Job drawing, mm, ordinate dimensions from the low corner. One solid piece. Give positions to 0.01 mm unless a question says otherwise; leave off trailing zeros. Write each loop counter-clockwise with the first axis right and the second up, starting at its lowest first coordinate (ties: lowest second). Pieces come first, ordered by that corner, then holes. Notation, with made-up numbers: (1, 81.5) - (51, 81.5) arc R26 cw to (51, 110.5) - close; hole circle Ø3 at (55.25, 32). An arc over 180 degrees is marked (long way). Answer as a JSON object with one key per item and string values.
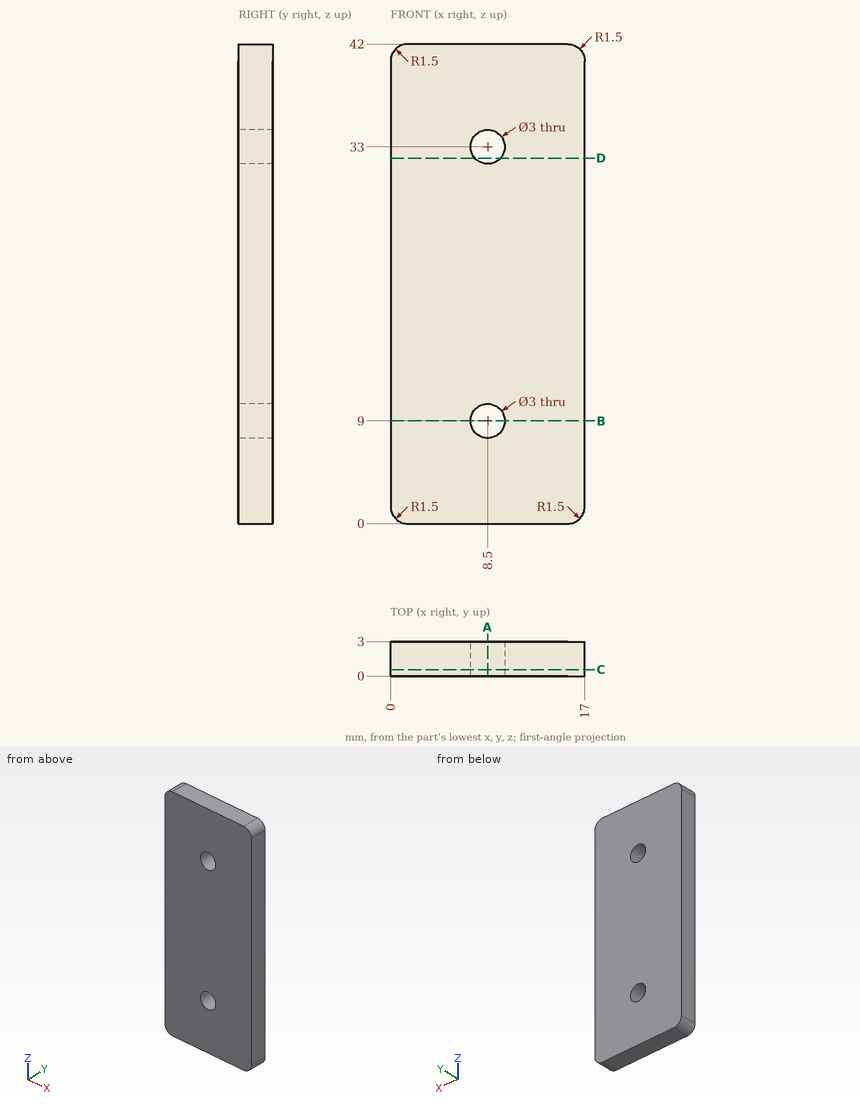
Item 1: Cut at A-A (x = 8.5). Give the cut face in (y, z), and give its area (3 significant figures).
Entries:
{"outline": "(0, 0) - (3, 0) - (3, 7.5) - (0, 7.5) - close; (0, 10.5) - (3, 10.5) - (3, 31.5) - (0, 31.5) - close; (0, 34.5) - (3, 34.5) - (3, 42) - (0, 42) - close", "area": "108 mm2"}
Item 2: Flat gauge pins, fed straight in: P1, Ø5, axis at x = 8.5, z = 9, coming from the +Y side; P2, Ø2.5, axis at x = 8.5, z = 33, coming from the -Y side. Where does each tip first touch, or does it go through?
Entries:
{"P1": "y = 3", "P2": "through"}
Item 3: Cut at D-D (z = 32). Give the cut face in (x, y), and give its area (3 significant figures).
Entries:
{"outline": "(0, 0) - (7.38, 0) - (7.38, 3) - (0, 3) - close; (9.62, 0) - (17, 0) - (17, 3) - (9.62, 3) - close", "area": "44.3 mm2"}
Item 4: Probe line 1 (Z direction, x = 8.5, y = 2); line 2 (Z direction, x = 9, y = 1.7); line 3 (X direction, y = 2.85, z = 8.5). List the from-to ranges inside material, lowest first. Write a range as from..to.
Entries:
{"line 1": "0..7.5, 10.5..31.5, 34.5..42", "line 2": "0..7.59, 10.41..31.59, 34.41..42", "line 3": "0..7.09, 9.91..17"}
Item 5: Cut at C-C (y = 0.55). Give the cut face in (x, z), and give its area (3 significant figures).
Entries:
{"outline": "(0, 1.5) arc R1.5 ccw to (1.5, 0) - (15.5, 0) arc R1.5 ccw to (17, 1.5) - (17, 40.5) arc R1.5 ccw to (15.5, 42) - (1.5, 42) arc R1.5 ccw to (0, 40.5) - close; hole circle Ø3 at (8.5, 9); hole circle Ø3 at (8.5, 33)", "area": "698 mm2"}
Item 6: Cut at B-B (z = 9). Give the cut face in (x, y).
Entries:
{"outline": "(0, 0) - (7, 0) - (7, 3) - (0, 3) - close; (10, 0) - (17, 0) - (17, 3) - (10, 3) - close"}
